```python
from build123d import *


with BuildPart() as part:
    # Sketch → Revolution (revolve)
    with BuildSketch(Plane.XY):
        with BuildLine():
            Line((10, 0), (12, 0))
            Line((12, 0), (12, 6.403799))
            ThreePointArc((13.070912, 9.18364), (12.276986, 7.893293), (12, 6.403799))
            Line((13.070912, 9.18364), (50, 50))
            Line((50, 50), (48.730875, 50))
            ThreePointArc((48.730875, 50), (48.062831, 49.858422), (47.509646, 49.45803))
            Line((47.509646, 49.45803), (11.078349, 9.19186))
            ThreePointArc((11.078349, 9.19186), (10.27891, 7.892552), (10, 6.392715))
            Line((10, 6.392715), (10, 0))
        make_face()
    revolve(axis=Axis((0, 0, 0), (0, 1, 0)))


solid = part.part
```
For this review, take the finished solid that the model builds, in its own axes (mm). A direction names the side the tool comes from. Coordinates: 2 decimals unless noted, no trailing zeros. Write each loop counter-clockwise with the first axis right and the second up, starting at its lowest first coordinate (ties: lowest second). Pieces come first, ordered by that corner, then holes.
(1) Add section C-C on y = 27. Give the boundary of the cut face in (x, z).
(2) Add section D-D on y = 12.5. Give the boundary of the cut face in (x, z), then the cut area to 3 significant figures.
(3) Add section B-B on z = 0. Give the boundary of the cut face in (x, y).
(4) Tool access review of faces 1 (the face through (48, 50, 11)), 2 (the face through (-11.99, 3.25, -0.53)): name each direction out of +Z, -Z, +X, -X, +Y, -Y from which nothing blocks a thin tool from reaching the whole face with its end or side.
(5) The part is to be moulded in two halves that separate along Z. For faces 3 (the face through (-2.17, 3.15, 9.76)), 4 (the face through (-4.22, 16.27, 19.02)), 5 (the face through (5, 0, -9)), say which applies: +Z half, -Z half, draft (parallel to the pull), parting line (faces both ways), or undercut.
(6) Wall thickness on probe 1 along Z at (x, y) = (0, 4); probe 2 along X at (y, z) = (36.5, -10): over which ranges is each line inside the solid? List them lowest first.
(7) For pin 1 Ø3 at (x, y) = (-0.5, 30.5) entering from -Z; pin 2 Ø1.5 at (y, z) = (38.5, 32) entering from -X; pin 3 Ø6 at (x, z) = (-23, 15) entering from -Y, all flat-tipped, find the tip position at first contact; note any pin that passes through.
(8) Add section A-A on x = 0. Give the boundary of the cut face in (y, z), then the cut area to 3 significant figures.
Answer sheet:
1. outline: circle Ø58.38 at (0, 0); hole circle Ø54.38 at (0, 0)
2. outline: circle Ø32.14 at (0, 0); hole circle Ø28.14 at (0, 0)
2. area: 189 mm2
3. outline: (-50, 50) - (-13.07, 9.18) arc R4.14 cw to (-12, 6.4) - (-12, 0) - (-10, 0) - (-10, 6.39) arc R4.17 ccw to (-11.08, 9.19) - (-47.51, 49.46) arc R1.65 ccw to (-48.73, 50) - close; (10, 0) - (12, 0) - (12, 6.4) arc R4.14 cw to (13.07, 9.18) - (50, 50) - (48.73, 50) arc R1.65 ccw to (47.51, 49.46) - (11.08, 9.19) arc R4.17 ccw to (10, 6.39) - close
4. face 1: +Z, -Z, +X, -X, +Y
4. face 2: -Y
5. face 3: undercut
5. face 4: parting line
5. face 5: draft
6. probe 1: z = -12 to -10, 10 to 12
6. probe 2: x = -36.44 to -34.36, 34.36 to 36.44
7. pin 1: stops at z = -33.71
7. pin 2: stops at x = -24.82
7. pin 3: stops at y = 21.77
8. outline: (0, -12) - (6.4, -12) arc R4.14 cw to (9.18, -13.07) - (50, -50) - (50, -48.73) arc R1.65 ccw to (49.46, -47.51) - (9.19, -11.08) arc R4.17 ccw to (6.39, -10) - (0, -10) - close; (0, 10) - (6.39, 10) arc R4.17 ccw to (9.19, 11.08) - (49.46, 47.51) arc R1.65 ccw to (50, 48.73) - (50, 50) - (9.18, 13.07) arc R4.14 cw to (6.4, 12) - (0, 12) - close
8. area: 200 mm2
